from build123d import *
from build123d import SkipClean  # not in build123d's __all__

# Parameters (mm, degrees)
F1_DEPTH = 25
F3_R     = 2


with BuildPart() as f1:
    # F0 (on Top) → F1 (new body)
    with BuildSketch(Plane.XY):
        with BuildLine():
            ThreePointArc((140, 36), (121, 55), (140, 74))
            Line((140, 74), (140, 96.25))
            ThreePointArc((140, 96.25), (128.4866545127, 94.6106724973), (117.8884190329, 89.8229879123))
            ThreePointArc((117.8884190329, 89.8229879123), (81.203397703, 82.0861941742), (48.4444483171, 100.3207767702))
            ThreePointArc((48.4444483171, 100.3207767702), (18.0058525586, 108.309129477), (0, 82.5))
            Line((0, 82.5), (0, 60))
            ThreePointArc((0, 60), (7.7212902527, 66.0859717551), (8.3025905106, 75.9002198354))
            ThreePointArc((8.3025905106, 75.9002198354), (29.5840689899, 102.832362125), (43.2539034221, 71.3462184874))
            ThreePointArc((43.2539034221, 71.3462184874), (30.1846255305, 51.9598971701), (18.2558114501, 31.8517179024))
            ThreePointArc((18.2558114501, 31.8517179024), (25.8689742306, 17.0641668337), (36.6109152463, 29.7623012378))
            ThreePointArc((36.6109152463, 29.7623012378), (35.6652555644, 44.2047922692), (40.8124091235, 57.7320473369))
            ThreePointArc((40.8124091235, 57.7320473369), (47.7320473369, 59.1875908765), (49.1875908765, 52.2679526631))
            ThreePointArc((49.1875908765, 52.2679526631), (45.5543060113, 42.7193020271), (46.2218304926, 32.5246024755))
            ThreePointArc((46.2218304926, 32.5246024755), (24.7379484611, 7.1283336674), (9.5116229002, 36.7034358047))
            ThreePointArc((9.5116229002, 36.7034358047), (21.7349755999, 57.308113326), (35.1269517111, 77.1731092437))
            ThreePointArc((35.1269517111, 77.1731092437), (28.2920344949, 92.9161810625), (17.6512952553, 79.4501099177))
            ThreePointArc((17.6512952553, 79.4501099177), (16.3752735006, 61.1617226531), (1.6270466845, 50.2721337703))
            ThreePointArc((1.6270466845, 50.2721337703), (0.8248238755, 50.0685027046), (0, 50))
            Line((0, 50), (0, 27.5))
            ThreePointArc((0, 27.5), (18.0058525586, 1.690870523), (48.4444483171, 9.6792232298))
            ThreePointArc((48.4444483171, 9.6792232298), (81.203397703, 27.9138058258), (117.8884190329, 20.1770120877))
            ThreePointArc((117.8884190329, 20.1770120877), (128.4866545127, 15.3893275027), (140, 13.75))
            Line((140, 13.75), (140, 36))
        make_face()
    extrude(amount=F1_DEPTH)

    # F2: F1 across face


with BuildPart() as f1_1:
    add(f1.part, clean=False)
    with SkipClean():  # cleaning this boolean's faces spoils the solid; the shape is the same uncleaned
        add(f1.part.mirror(Plane(origin=(140, 85.125, 12.5), x_dir=(0, 1, 0), z_dir=(1, 0, 0))), clean=False)

    # F3
    f3_edges = [f1_1.edges().sort_by_distance(p)[0] for p in [
        (0, 60, 12.5),
        (0, 50, 12.5),
        (280, 60, 12.5),
        (280, 50, 12.5),
    ]]
    fillet(f3_edges, radius=F3_R)


solid = f1_1.part
Input: part model. Units: mm. Frame: model coordinates. A direction names the side the tool comes from. Coordinates: 2 decimals unless noted, no trailing zeros. Loops run counter-clockwise (first coordinate to the right, second up) from the corner with the lowest first, then second, coordinate; pieces in that order, holes last. Notation, with made-up numbers: (14, -21.75) -> (60, -21.75) arc R19 cw to (60, -16.75) -> close; hole circle Ø2 at (46.25, 88.5). An arc over 180 degrees is marked (long way). Write each question's results on one line, items separated by ' | '. Start each with the question number.
Q1. Reachability of faces 4 (the cylindrical face through (262.433, 1.857, 12.325)), 5 (the cylindrical face through (30.36, 52.24, 12.32)) from +Z, -Z, +X, -X, +Y, -Y: full face, straight path, thin tool, end or side. Return the list, or none.
Q2. Ray query, line 1 (X direction, y = 47, z = 4.5); line 2 (X direction, y = 67.5, z = 3); line 3 (Y direction, x = 27, z = 6). Return the intervals inside material, ascending. Write a range as from..to.
Q3. Pull-direction query (X, two-part tool) for faces 1 (the flat face through (280, 73, 12)), 2 (the flat face through (0, 73, 12)), 3 (the cylindrical face through (198.27, 82.01, 12.32)); classes: released by +X, released by -X, zero draft, split by the parting line, or undercut.
Q4. Pin query (flat end, axial travel): pin 1 (2 mm diameter, centred on x = 123, z = 12.5, fed in from -Y); pin 2 (1.5 mm diameter, centred on x = 148, y = 75, fed in from -Z); pin 3 (4 mm diameter, centred on x = 178.5, z = 11, fed in from +Y); pin 4 (1 mm diameter, centred on y = 14, z = 20.5, fed in from -X). Return the tip coordinate at first contact, or that it passes through.
Q5. Section D-D, the plane x = 202.5. Return the cut outline in (y, z).
Q6. Section B-B, the plane x = 253. Return the cut outline in (y, z).
Q7. Section A-A, the plane y = 55. Return the cut outline in (x, z).
Q8. Section C-C, the plane y = 40. Return the cut outline in (x, z), plus the area to 3 significant figures.
Found:
1) face 4: +Z, -Z, -Y | face 5: +Z, -Z
2) line 1: 0..15.42, 27.1..36.21, 46.61..122.77, 157.23..233.39, 243.79..252.9, 264.58..280 | line 2: 0..8.35, 18.67..28.4, 40.53..125.69, 154.31..239.47, 251.6..261.33, 271.65..280 | line 3: 0..7, 17..46.84, 65.42..93, 103..110
3) face 1: released by +X | face 2: released by -X | face 3: undercut
4) pin 1: y = 16.98 | pin 2: z = 0 | pin 3: y = 83.43 | pin 4: x = 3.27
5) outline: (27.22, 0) -> (82.78, 0) -> (82.78, 25) -> (27.22, 25) -> close
6) outline: (0, 0) -> (7, 0) -> (7, 25) -> (0, 25) -> close; (17, 0) -> (46.84, 0) -> (46.84, 25) -> (17, 25) -> close; (65.42, 0) -> (93, 0) -> (93, 25) -> (65.42, 25) -> close; (103, 0) -> (110, 0) -> (110, 25) -> (103, 25) -> close
7) outline: (11.34, 0) -> (20.28, 0) -> (20.28, 25) -> (11.34, 25) -> close; (32.13, 0) -> (39.21, 0) -> (39.21, 25) -> (32.13, 25) -> close; (50, 0) -> (121, 0) -> (121, 25) -> (50, 25) -> close; (159, 0) -> (230, 0) -> (230, 25) -> (159, 25) -> close; (240.79, 0) -> (247.87, 0) -> (247.87, 25) -> (240.79, 25) -> close; (259.72, 0) -> (268.66, 0) -> (268.66, 25) -> (259.72, 25) -> close
8) outline: (0, 0) -> (11.36, 0) -> (11.36, 25) -> (0, 25) -> close; (22.9, 0) -> (35.3, 0) -> (35.3, 25) -> (22.9, 25) -> close; (45.3, 0) -> (128.34, 0) -> (128.34, 25) -> (45.3, 25) -> close; (151.66, 0) -> (234.7, 0) -> (234.7, 25) -> (151.66, 25) -> close; (244.7, 0) -> (257.1, 0) -> (257.1, 25) -> (244.7, 25) -> close; (268.64, 0) -> (280, 0) -> (280, 25) -> (268.64, 25) -> close | area: 5,340 mm2
